The listing builds one solid part. Answer for the finished solid, in the listing's coordinates (mm). A direction names the side the tool comes from. Coordinates: 2 decimals unless noted, no trailing zeros. Write each loop counter-clockwise with the first axis right and the second up, starting at its lowest first coordinate (ties: lowest second). Pieces come first, ordered by that corner, then holes.
(1) Given P1, Ø2, axis at y = 10, z = 5.5, coming from the +X side; P2, Ø7.5, axis at x = -34.38, y = 15.33, coming from the -Z side; P3, Ø12, axis at x = -56.5, z = 13.5, coming from the -Y side; P4, Ø8, axis at y = 13.5, z = 19.5, coming from the +X side, each flat-ended and moving along its own axis, determine where each tip first touches the part or whether it passes through.
(2) For a pull along X with two mould halves and no side action, classify faces 4 (the flat face through (-30, 7.27, 21.31)), 5 (the flat face through (-21.53, 8.54, 11.47)), 6 (the flat face through (-47.82, 16.07, 20.04)), 7 (the cylindrical face through (-20.325, 32.153, 27.492)) as +X half, -X half, draft (parallel to the pull), parting line (faces both ways), or undercut.
(3) The part is cut by section D-D on z = 25.5. Determine the outline of the cut face in (x, y), plus the area to 3 significant figures.
(4) The part is cut by section A-A on x = -57.15. Determine the outline of the cut face in (y, z), plus the area to 3 significant figures.
(5) Which of the six approach directions +Z, -Z, +X, -X, +Y, -Y give full straight-line access (tool end or side, diameter ignored) to faces 1 (the cylindrical face through (-29.32, 8.74, 27.49)), 2 (the cylindrical face through (-0.764, 50.076, 20.604)), 3 (the flat face through (-30.016, 5.455, 20.135))?
(6) Straight lines are drawn through the part: line 1 (Y direction, x = -25.4, z = 2.75); line 2 (X direction, y = 44, z = 17); line 3 (Y direction, x = -30, z = 33). For each, find the intervals that lie inside material, in ascending order.
(7) The part is cut by section C-C on z = 10. Determine the outline of the cut face in (x, y) (3 decimals).
(8) The part is cut by section B-B on y = 44.45. Determine the outline of the cut face in (x, z).
from build123d import *

# Parameters (mm, degrees)
SKETCH1_R           = 2.286
BOSS_EXTRUDE1_DEPTH = 40.64
SKETCH2_R           = 41.91
CUT_EXTRUDE1_DEPTH  = 26.67
SKETCH3_R           = 29.21
CUT_EXTRUDE2_DEPTH  = 91.909293254
SKETCH4_R           = 2.286
CUT_EXTRUDE3_DEPTH  = 91.909293254
CUT_EXTRUDE4_DEPTH  = 31.75
FILLET1_R           = 6.35
FILLET2_R           = 2.54
FILLET3_R           = 6.35


with BuildPart() as part:
    # Sketch1 → Boss-Extrude1 (new body)
    with BuildSketch(Plane.XY):
        Polygon((-63.5, 31.75), (-31.75, 0), (0, 0), (0, 50.8), (-63.5, 50.8), align=None)
        with Locations((-57.15, 44.45)):
            Circle(SKETCH1_R, mode=Mode.SUBTRACT)
        with Locations((-19.091771775, 44.45)):
            Circle(SKETCH1_R, mode=Mode.SUBTRACT)
        with Locations((-34.380256121, 15.330256121)):
            Circle(SKETCH1_R, mode=Mode.SUBTRACT)
    extrude(amount=BOSS_EXTRUDE1_DEPTH)

    # Sketch2 → Cut-Extrude1 (cut)
    with BuildSketch(Plane.XY.offset(40.64)):
        with Locations((12.7, 6.35)):
            Circle(SKETCH2_R)
    extrude(amount=-CUT_EXTRUDE1_DEPTH, mode=Mode.SUBTRACT)

    # Sketch3 → Cut-Extrude2 (cut, through all)
    with BuildSketch(Plane(origin=(0, 0, 0), x_dir=(-1, 0, 0), z_dir=(0, 0, -1))):
        with Locations((-12.7, 6.35)):
            Circle(SKETCH3_R)
    extrude(amount=-CUT_EXTRUDE2_DEPTH, mode=Mode.SUBTRACT)

    # Sketch4 → Cut-Extrude3 (cut, through all)
    with BuildSketch(Plane(origin=(0, 0, 0), x_dir=(-1, 0, 0), z_dir=(0, 0, -1))):
        with Locations((25.4, 6.35)):
            Circle(SKETCH4_R)
    extrude(amount=-CUT_EXTRUDE3_DEPTH, mode=Mode.SUBTRACT)

    # Sketch5 → Cut-Extrude4 (cut)
    with BuildSketch(Plane.XY.offset(40.64)):
        Polygon((-20.267356107, 6.35), (-22.833678053, 10.795), (-27.966321947, 10.795), (-30.532643893, 6.35), (-27.966321947, 1.905), (-22.833678053, 1.905), align=None)
    extrude(amount=-CUT_EXTRUDE4_DEPTH, mode=Mode.SUBTRACT)

    # Fillet1
    fillet1_edges = [part.edges().sort_by_distance(p)[0] for p in [
        (0, 32.654640275, 6.985),
        (-15.811429287, 0, 6.985),
        (-31.75, 0, 20.32),
        (-63.5, 31.75, 20.32),
    ]]
    fillet(fillet1_edges, radius=FILLET1_R)

    # Fillet2
    fillet2_edges = [part.edges().sort_by_distance(p)[0] for p in [
        (0, 46.289430392, 27.305),
        (0, 50.8, 20.32),
    ]]
    fillet(fillet2_edges, radius=FILLET2_R)

    # Fillet3
    fillet3_edges = [part.edges().sort_by_distance(p)[0] for p in [
        (-29.140585836, 3.938884718, 27.305),
        (-29.140585836, 8.761115282, 27.305),
    ]]
    fillet(fillet3_edges, radius=FILLET3_R)


solid = part.part
Model answer:
1. P1: stops at x = -16.14
1. P2: stops at z = 0
1. P3: stops at y = 18.75
1. P4: stops at x = -27.7
2. face 4: undercut
2. face 5: undercut
2. face 6: -X half
2. face 7: +X half
3. outline: (-63.5, 34.38) arc R6.35 ccw to (-61.64, 29.89) - (-33.61, 1.86) arc R6.35 ccw to (-29.12, 0) - (-28.73, 0) arc R41.91 cw to (-29.04, 2.59) arc R6.35 ccw to (-29.87, 5.2) - (-30.53, 6.35) - (-29.87, 7.5) arc R6.35 ccw to (-29.04, 10.11) arc R41.91 cw to (-1.67, 45.72) arc R2.54 ccw to (0, 48.11) - (0, 48.26) arc R2.54 ccw to (-2.54, 50.8) - (-63.5, 50.8) - close; hole circle Ø4.57 at (-57.15, 44.45); hole circle Ø4.57 at (-34.38, 15.33); hole circle Ø4.57 at (-19.09, 44.45)
3. area: 1,630 mm2
4. outline: (25.4, 0) - (42.16, 0) - (42.16, 40.64) - (25.4, 40.64) - close; (46.74, 0) - (50.8, 0) - (50.8, 40.64) - (46.74, 40.64) - close
4. area: 846 mm2
5. face 1: +Z, +X
5. face 2: +Z, -Z, +X, +Y
5. face 3: +Z
6. line 1: y = 0 to 4.06, 8.64 to 50.8
6. line 2: x = -63.5 to -59.39, -54.91 to -21.33, -16.85 to -5.71
6. line 3: y = 0.06 to 5.43, 7.27 to 50.8
7. outline: (-63.5, 34.38) arc R6.35 ccw to (-61.64, 29.89) - (-33.61, 1.86) arc R6.35 ccw to (-29.12, 0) - (-22.86, 0) arc R6.35 ccw to (-16.51, 6.35) arc R29.21 cw to (-2.948, 31.015) arc R6.35 ccw to (0, 36.377) - (0, 48.26) arc R2.54 ccw to (-2.54, 50.8) - (-63.5, 50.8) - close; hole circle Ø4.572 at (-57.15, 44.45); hole circle Ø4.572 at (-34.38, 15.33); hole (-30.533, 6.35) - (-27.966, 1.905) - (-22.834, 1.905) - (-20.267, 6.35) - (-22.834, 10.795) - (-27.966, 10.795) - close; hole circle Ø4.572 at (-19.092, 44.45)
8. outline: (-63.5, 0) - (-59.44, 0) - (-59.44, 40.64) - (-63.5, 40.64) - close; (-54.86, 0) - (-21.38, 0) - (-21.38, 40.64) - (-54.86, 40.64) - close; (-16.81, 0) - (0, 0) - (0, 13.97) - (-4.76, 13.97) - (-4.76, 40.64) - (-16.81, 40.64) - close
